Source: CAD feature listing. Evaluate the final solid. Frame: model axes, mm. A direction names the side the tool comes from. Round coordinates to 2 decimals unless told otherwise and drop trailing zeros. Loops run counter-clockwise (first coordinate to the right, second up) from the corner with the lowest first, then second, coordinate; pieces in that order, holes last.
(1) Set-up query: faces 1 (the cylindrical face through (13, 2, 0)), 2 (the flat face through (1.5, 3, 1.8)). Return all of +Z, -Z, +X, -X, +Y, -Y with unobstructed straight access to the full face (end or side cutting, diameter ignored); none if empty.
(2) Material intervals for probe 1 along X at (y, z) = (0.25, 1.25) (3 decimals); probe 2 along X at (y, z) = (2, -2.25) (3 decimals); probe 3 along Y at (x, z) = (0.2, 0), sorted ascending.
(3) Section A-A, the plane x = 2.75. Return the cut outline in (y, z), plus the area to 3 significant figures.
(4) First-contact query: pin 1 Ø1 at (y, z) = (3, 0) entering from +X. Flat tip, straight axial feed; report the tip coordinate or a pass-through.
(5) Mould query, pull axis Y, two halves, no side actions, for faces 3 (the cylindrical face through (0.18, 2.58, -1.65)), 4 (the flat face through (1.479, 3.045, -1.726)), 5 (the flat face through (1.5, -3, -1.8)), 6 (the flat face through (0.375, 0, 0)). Classes: pulls with the +Y half, pulls with the -Y half, needs draft (parallel to the pull), parting line crosses it, or undercut.
```python
from build123d import *

# Parameters (mm, degrees)
SKETCH2_R     = 4.081986143
HEX_DIE_DEPTH = 3
SKETCH4_R     = 3.0625
INDENT_DEPTH  = 0.375


with BuildPart() as part:
    # BodySke → Base-Revolve (revolve)
    with BuildSketch(Plane.XY, mode=Mode.PRIVATE) as base_revolve_sk:
        Polygon((3, 2), (3, 4.041570439), (0.312675839, 4.041570439), (0, 3.5), (0, 0), (23, 0), (23, 2), align=None)
    revolve(base_revolve_sk.sketch.rotate(Axis((-25.4, 0, 0), (1, 0, 0)), 90), axis=Axis((-25.4, 0, 0), (1, 0, 0)))

    # Sketch2 → Hex-Die (cut)
    with BuildSketch(Plane(origin=(0, 0, 0), x_dir=(0, 0, -1), z_dir=(1, 0, 0))):
        Circle(SKETCH2_R)
        Polygon((-3.5, 2.020725951), (0, 4.041451902), (3.5, 2.020725951), (3.5, -2.020725951), (0, -4.041451902), (-3.5, -2.020725951), align=None, mode=Mode.SUBTRACT)
    extrude(amount=HEX_DIE_DEPTH, mode=Mode.SUBTRACT)

    # Sketch4 → Indent (cut)
    with BuildSketch(Plane(origin=(0, 0, 0), x_dir=(0, 0, -1), z_dir=(1, 0, 0))):
        Circle(SKETCH4_R)
    extrude(amount=INDENT_DEPTH, mode=Mode.SUBTRACT)


solid = part.part
```
Output values:
1. face 1: +X
1. face 2: +Z, +X, -X, +Y
2. probe 1: x = 0.375 to 23
2. probe 2: x = 0.375 to 3
2. probe 3: y = -3.85 to -3.06, 3.06 to 3.85
3. outline: (-4.04, 0) - (-2.02, -3.5) - (2.02, -3.5) - (4.04, 0) - (2.02, 3.5) - (-2.02, 3.5) - close
3. area: 42.4 mm2
4. pin 1: stops at x = 3
5. face 3: undercut
5. face 4: pulls with the +Y half
5. face 5: pulls with the -Y half
5. face 6: undercut
